Design review of the part built by this model. Coordinates are the model's own, in mm. Coordinates: 2 decimals unless noted, no trailing zeros. Write each loop counter-clockwise with the first axis right and the second up, starting at its lowest first coordinate (ties: lowest second). Pieces come first, ordered by that corner, then holes.
Q1. The part is to be moulded in two halves that separate along X. For faces 1 (the cylindrical face through (-2.694, 0.986, -74.235)), 2 (the flat face through (-152.26, 0.99, -73.48)), 3 (the flat face through (-79, 0, -39)), say which applies: released by +X, released by -X, zero draft, split by the parting line, or undercut.
Q2. For L1, parallel to Z at x = -3.5, y = 1.65; L2, parallel to X at y = 0.75, z = -3.5, list the stretches that pass through material, from the lowest coordinate up.
Q3. Take a section at A-A, the plane z = -3.5. Write out the cut boundary in (x, y), plus the area to 3 significant figures.
Q4. Take a section at B-B, the plane x = -3.5. Write out the cut boundary in (y, z), plus the area to 3 significant figures.
from build123d import *

# Parameters (mm, degrees)
SKETCH2_R           = 1.5
BOSS_EXTRUDE1_DEPTH = 2


with BuildPart() as part:
    # Sketch2 → Boss-Extrude1 (new body)
    with BuildSketch(Plane(origin=(0, 0, 0), x_dir=(1, 0, 0), z_dir=(0, 1, 0))):
        Polygon((-149.27, 76.47), (-155.34404725, 70.39595275), (-155.34404725, 6.07404725), (-149.27, 0), (0, 0), (0, 76.47), align=None)
        with Locations((-3.5, 72.97)):
            Circle(SKETCH2_R, mode=Mode.SUBTRACT)
        with Locations((-3.5, 3.5)):
            Circle(SKETCH2_R, mode=Mode.SUBTRACT)
        with Locations((-145.77, 72.97)):
            Circle(SKETCH2_R, mode=Mode.SUBTRACT)
        with Locations((-145.77, 3.5)):
            Circle(SKETCH2_R, mode=Mode.SUBTRACT)
    extrude(amount=BOSS_EXTRUDE1_DEPTH)


solid = part.part
Responses:
1. face 1: undercut
1. face 2: released by -X
1. face 3: zero draft
2. L1: z = -76.47 to -74.47, -71.47 to -5, -2 to 0
2. L2: x = -152.77 to -147.27, -144.27 to -5, -2 to 0
3. outline: (-152.77, 0) - (-147.27, 0) - (-147.27, 2) - (-152.77, 2) - close; (-144.27, 0) - (-5, 0) - (-5, 2) - (-144.27, 2) - close; (-2, 0) - (0, 0) - (0, 2) - (-2, 2) - close
3. area: 294 mm2
4. outline: (0, -76.47) - (2, -76.47) - (2, -74.47) - (0, -74.47) - close; (0, -71.47) - (2, -71.47) - (2, -5) - (0, -5) - close; (0, -2) - (2, -2) - (2, 0) - (0, 0) - close
4. area: 141 mm2
